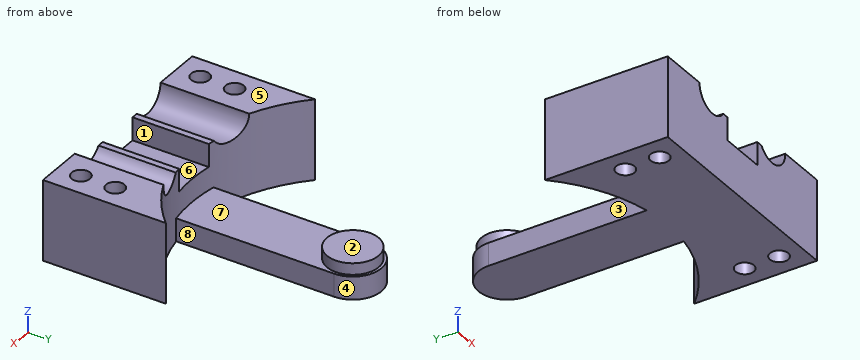
from build123d import *

# Parameters (mm, degrees)
BOSS_EXTRUDE1_DEPTH = 7
BOSS_EXTRUDE2_DEPTH = 2
BOSS_EXTRUDE3_START = 2
SKETCH3_R           = 2.25
BOSS_EXTRUDE3_DEPTH = 1
SKETCH4_R           = 0.8
SCREW_HOLES_DEPTH   = 8
CABLE_START         = -20.5
SKETCH6_R           = 1.75
CABLE_TUBES_DEPTH   = 18.5
WIRE_START          = -20.5
WIRE_CANALS_DEPTH   = 7.5


with BuildPart() as part:
    # Sketch1 → Boss-Extrude1 (new body)
    with BuildSketch(Plane.XY):
        with BuildLine():
            ThreePointArc((10, -9.797958971), (0, -14), (-10, -9.797958971))
            Line((-10, -9.797958971), (-10, -20.5))
            Line((-10, -20.5), (10, -20.5))
            Line((10, -20.5), (10, -9.797958971))
        make_face()
    extrude(amount=BOSS_EXTRUDE1_DEPTH)

    # Sketch2 → Boss-Extrude2 (add)
    with BuildSketch(Plane.XY):
        with BuildLine():
            Line((-2.5, 0), (-2.5, -20.5))
            Line((-2.5, -20.5), (2.5, -20.5))
            Line((2.5, -20.5), (2.5, 0))
            ThreePointArc((2.5, 0), (0, 2.5), (-2.5, 0))
        make_face()
    extrude(amount=BOSS_EXTRUDE2_DEPTH)

    # Sketch3 → Boss-Extrude3 (add)
    with BuildSketch(Plane.XY.offset(BOSS_EXTRUDE3_START)):
        Circle(SKETCH3_R)
    extrude(amount=BOSS_EXTRUDE3_DEPTH)

    # Sketch4 → Screw Holes (cut, through all)
    with BuildSketch(Plane.XY):
        with Locations((-8, -15.5)):
            Circle(SKETCH4_R)
        with Locations((8, -15.5)):
            Circle(SKETCH4_R)
        with Locations((-8, -18.5)):
            Circle(SKETCH4_R)
        with Locations((8, -18.5)):
            Circle(SKETCH4_R)
    extrude(amount=SCREW_HOLES_DEPTH, mode=Mode.SUBTRACT)

    # Sketch6 → Cable Tubes (cut)
    with BuildSketch(Plane(origin=(0, 0, 0), x_dir=(1, 0, 0), z_dir=(0, 1, 0)).offset(CABLE_START)):
        with Locations((-4, -7)):
            Circle(SKETCH6_R)
        with Locations((4, -7)):
            Circle(SKETCH6_R)
    extrude(amount=CABLE_TUBES_DEPTH, mode=Mode.SUBTRACT)

    # Sketch7 → Wire Canals (cut)
    with BuildSketch(Plane(origin=(0, 0, 0), x_dir=(1, 0, 0), z_dir=(0, 1, 0)).offset(WIRE_START)):
        Polygon((-3, -6), (-2, -6), (-2, -4), (2, -4), (2, -6), (3, -6), (3, -7), (-3, -7), align=None)
    extrude(amount=WIRE_CANALS_DEPTH, mode=Mode.SUBTRACT)


solid = part.part
Can you work these out from the model? Positions are in its coordinate system, mm. Face numbers are marked on the shaded views. A direction names the side the tool comes from. Give positions to 0.01 mm unless a question says otherwise; leave off trailing zeros. Order: outer loops, then holes, each group sorted by start corner. A loop starts at its lowest first (then second) coordinate and runs counter-clockwise, first axis right, second up. Notation, with made-up numbers: M 40,42 L 84,42 A12 cw 84,60 Z; hole C -27,80.5 d6. An arc over 180 degrees is marked long. Use a Markdown table: item, result. Add a question column.
Item 1: Suppose I cut it at C-C (x = -8). List the corners of the cut face in (y, z) for me, then the cut area to 3 significant figures.
Item 2: Will these pins go through, and if not, where does the flat tip stop? pin 1 (3.5 mm diameter, centred on x = 0.5, y = 0.5, fed in from +Z); pin 2 (4 mm diameter, centred on x = -1, y = -9.5, fed in from +Z); pin 3 (0.6 mm diameter, centred on y = -5, z = 1, fed in from -X); pin 4 (1.8 mm diameter, centred on x = 8, y = -15.5, fed in from +Z).
Item 3: For the marked faces 5, 6, 7 and 8, which set-ups out of +Z, -Z, +X, -X, +Y, -Y let a thin tool reach every point of the face, with its end or its side?
Item 4: Suppose I cut it at A-A (y = -18.5). List the corners of the cut face in (x, z) for me.
Item 5: If I drill on L1, parallel to X at y = -15.5, z = 1.5; L2, parallel to Y at x = -8, z = 2; L3, parallel to X at y = -16, z = 5, over which ranges is the centre line in solid material (lowest first)? Write a range as [from, to].
Item 6: Suppose I cut it at D-D (x = 0). List the corners of the cut face in (y, z) for me, then the cut area to 3 significant figures.
Item 7: We'd pull the mould along X, two halves only. Please class the marked faces 1, 2, 3 and 4: +X half, -X half, draft (parallel to the pull), parting line (faces both ways), or undercut.
Item 8: Suppose I cut it at B-B (z = 1.5). List the corners of the cut face in (x, y) for me.
Answer sheet:
| question | item | result |
|---|---|---|
| 1 | outline | M -20.5,0 L -19.3,0 L -19.3,7 L -20.5,7 Z; M -17.7,0 L -16.3,0 L -16.3,7 L -17.7,7 Z; M -14.7,0 L -11.49,0 L -11.49,7 L -14.7,7 Z |
| 1 | area | 40.7 mm² |
| 2 | pin 1 | stops at z = 3 |
| 2 | pin 2 | stops at z = 2 |
| 2 | pin 3 | stops at x = -2.5 |
| 2 | pin 4 | stops at z = 7 |
| 3 | face 5 | +Z, +X, -X, +Y, -Y |
| 3 | face 6 | +Z, +Y, -Y |
| 3 | face 7 | +Z |
| 3 | face 8 | +Z, -Z, +Y |
| 4 | outline | M -10,0 L -8.8,0 L -8.8,7 L -10,7 Z; M -7.2,0 L 7.2,0 L 7.2,7 L 5.75,7 A1.75 cw 2.56,6 L 2,6 L 2,4 L -2,4 L -2,6 L -2.56,6 A1.75 cw -5.75,7 L -7.2,7 Z; M 8.8,0 L 10,0 L 10,7 L 8.8,7 Z |
| 5 | L1 | x = [-10, -8.8], [-7.2, 7.2], [8.8, 10] |
| 5 | L2 | y = [-20.5, -19.3], [-17.7, -16.3], [-14.7, -11.49] |
| 5 | L3 | x = [-10, -8.62], [-7.38, -2], [2, 7.38], [8.62, 10] |
| 6 | outline | M -20.5,0 L 2.5,0 L 2.5,2 L 2.25,2 L 2.25,3 L -2.25,3 L -2.25,2 L -14,2 L -14,4 L -20.5,4 Z |
| 6 | area | 63.5 mm² |
| 7 | face 1 | undercut |
| 7 | face 2 | draft |
| 7 | face 3 | undercut |
| 7 | face 4 | parting line |
| 8 | outline | M -10,-20.5 L 10,-20.5 L 10,-9.8 A14 cw 2.5,-13.77 L 2.5,0 A2.5 ccw -2.5,0 L -2.5,-13.77 A14 cw -10,-9.8 Z; hole C -8,-18.5 d1.6; hole C -8,-15.5 d1.6; hole C 8,-18.5 d1.6; hole C 8,-15.5 d1.6 |
